Answer from the drawing. Dimensions are ordinates in mm from the lowest x, y and z of the part. Give positions to 0.01 mm unless a question says otherwise; leave off trailing zeros. Loops run counter-clockwise (first coordinate to the right, second up) from the corner with the lowest first, then second, coordinate; pieces in that order, holes last. Notation, with made-up numbers: M 23,-13.5 L 61,-13.5 A19 ccw 61,21.5 Z; hole C 21,18 d11. An arc over 180 degrees is marked long. Return JSON: item names as keys, results as strings. Group by question number.
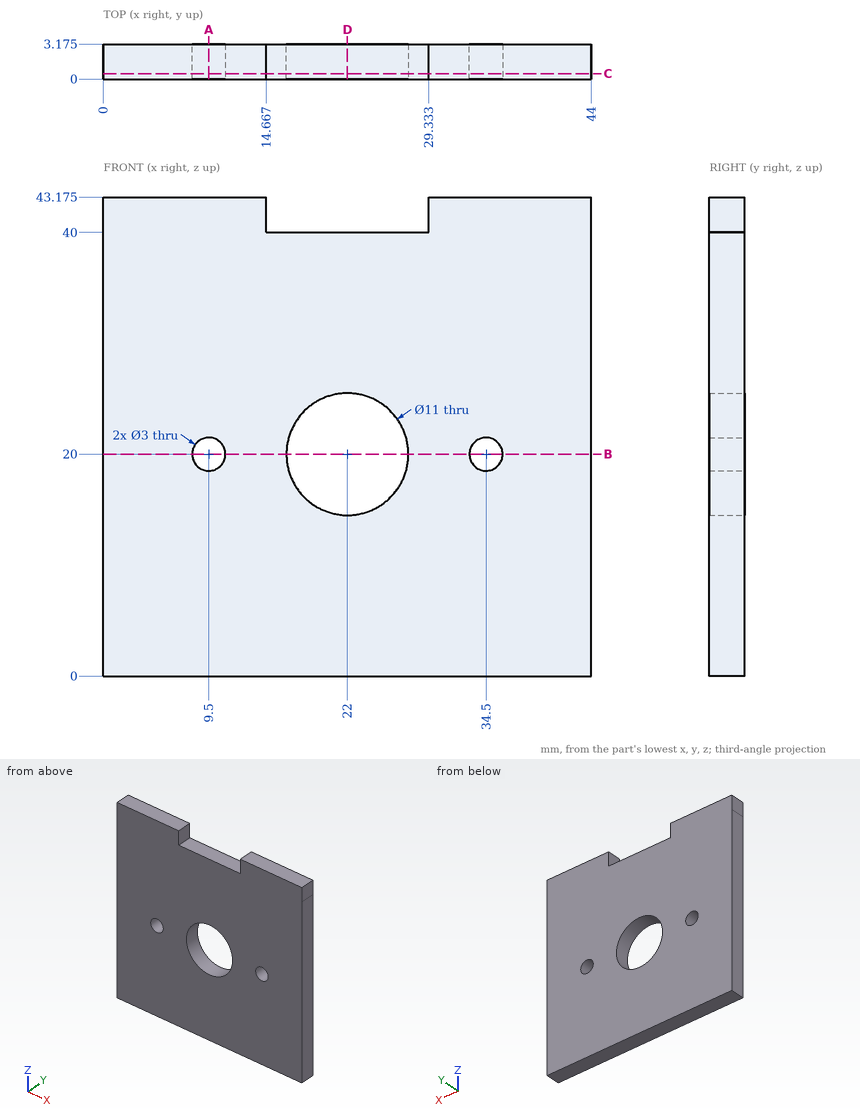
1. Straight lines are drawn through the part: line 1 along X through (y, z) = (1.85, 41); line 2 along X through (y, z) = (0.4, 17.5); line 3 along Z through (x, y) = (20.5, 0.45). For each, find the intervals that lie inside material, in ascending order.
2. Find section B-B (z = 20). Write down the section's boundary in (x, y) (1 decimal).
3. Find section A-A (x = 9.5). Write down the section's boundary in (y, z) (1 decimal).
4. Find section D-D (x = 22). Write down the section's boundary in (y, z) (1 decimal).
5. A flat-ended cylindrical pin translates along its axis: P1, Ø1, axis at x = 18.5, y = 1, coming from the +Z side. Find the tip coordinate at first contact, or state that the pin passes through.
6. Find section C-C (y = 0.5). Write down the section's boundary in (x, z) (1 decimal), and give its area (3 significant figures).
Result:
{
 "1": {"line 1": "x = 0 to 14.67, 29.33 to 44", "line 2": "x = 0 to 17.1, 26.9 to 44", "line 3": "z = 0 to 14.71, 25.29 to 40"},
 "2": {"outline": "M 0,0 L 8,0 L 8,3.2 L 0,3.2 Z; M 11,0 L 16.5,0 L 16.5,3.2 L 11,3.2 Z; M 27.5,0 L 33,0 L 33,3.2 L 27.5,3.2 Z; M 36,0 L 44,0 L 44,3.2 L 36,3.2 Z"},
 "3": {"outline": "M 0,0 L 3.2,0 L 3.2,18.5 L 0,18.5 Z; M 0,21.5 L 3.2,21.5 L 3.2,43.2 L 0,43.2 Z"},
 "4": {"outline": "M 0,0 L 3.2,0 L 3.2,14.5 L 0,14.5 Z; M 0,25.5 L 3.2,25.5 L 3.2,40 L 0,40 Z"},
 "5": {"P1": "stops at z = 40"},
 "6": {"outline": "M 0,0 L 44,0 L 44,43.2 L 29.3,43.2 L 29.3,40 L 14.7,40 L 14.7,43.2 L 0,43.2 Z; hole C 9.5,20 d3; hole C 22,20 d11; hole C 34.5,20 d3", "area": "1,740 mm2"}
}
